Can you work these out from the drawing? Everything is in mm from the part's minimum corner. Round coordinates to 2 decimals unless told otherwise and drop trailing zeros. Order: outer loops, then holes, each group sorted by start corner. A loop starts at its lowest first (then second) coordinate and runs counter-clockwise, first axis right, second up. Notation, with made-up numbers: (75.5, 85) -> (80.5, 85) arc R22 cw to (80.5, 115) -> close; hole circle Ø8 at (47, 56). An arc over 180 degrees is marked (long way). One line per item, written item: value.
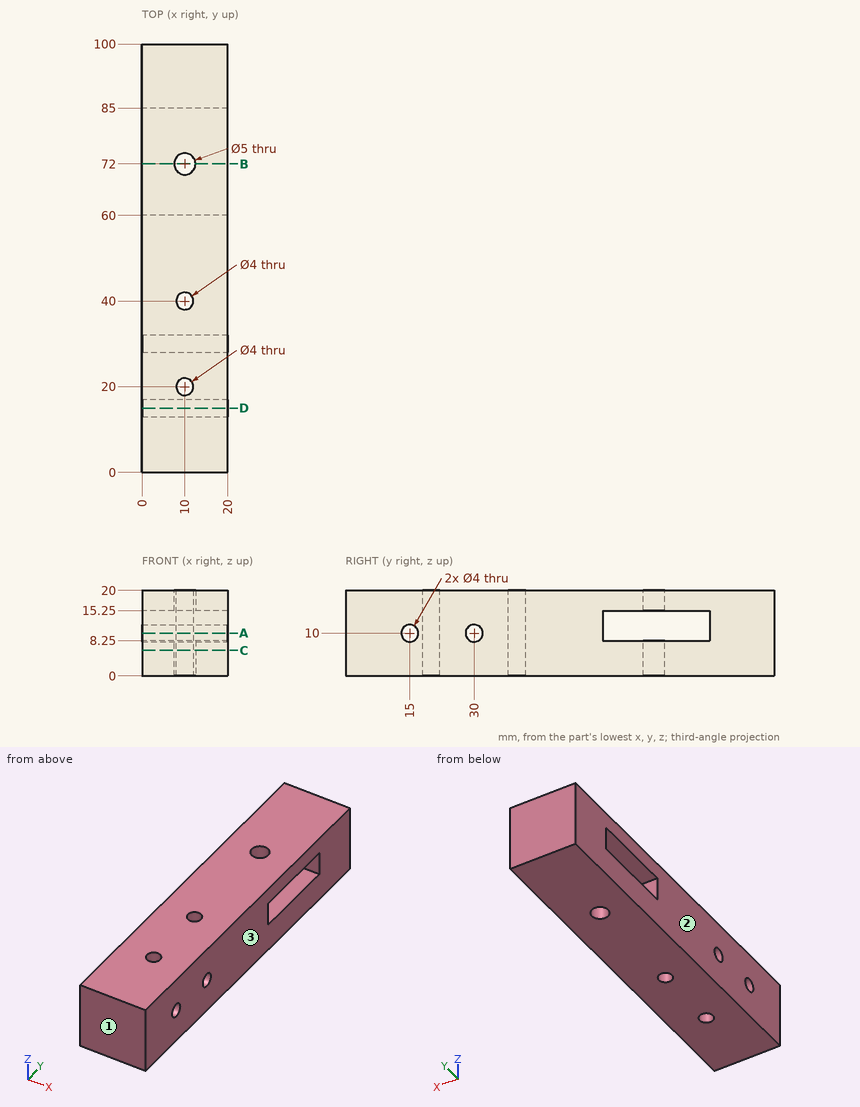
Q1. I want a section at A-A on z = 10. Write out the boundary of the cut face in (x, y).
Answers:
outline: (0, 0) -> (20, 0) -> (20, 13) -> (0, 13) -> close; (0, 17) -> (20, 17) -> (20, 28) -> (0, 28) -> close; (0, 32) -> (20, 32) -> (20, 60) -> (0, 60) -> close; (0, 85) -> (20, 85) -> (20, 100) -> (0, 100) -> close; hole circle Ø4 at (10, 20); hole circle Ø4 at (10, 40)
Q2. I want a section at B-B on y = 72. Write out the boundary of the cut face in (x, z).
Answers:
outline: (0, 0) -> (7.5, 0) -> (7.5, 8.25) -> (0, 8.25) -> close; (0, 15.25) -> (7.5, 15.25) -> (7.5, 20) -> (0, 20) -> close; (12.5, 0) -> (20, 0) -> (20, 8.25) -> (12.5, 8.25) -> close; (12.5, 15.25) -> (20, 15.25) -> (20, 20) -> (12.5, 20) -> close
Q3. I want a section at D-D on y = 15. Write out the boundary of the cut face in (x, z), then the cut area to 3 significant figures.
Answers:
outline: (0, 0) -> (20, 0) -> (20, 8) -> (0, 8) -> close; (0, 12) -> (20, 12) -> (20, 20) -> (0, 20) -> close
area: 320 mm2
Q4. I need wall thicknesses on line 1 along Y through (x, z) = (10, 14.5); line 2 along Y through (x, z) = (10, 17.1); line 3 along Z through (x, y) = (13.5, 15). Which ranges of each line are inside material? Lowest first, please.
Answers:
line 1: 0 to 18, 22 to 38, 42 to 60, 85 to 100
line 2: 0 to 18, 22 to 38, 42 to 69.5, 74.5 to 100
line 3: 0 to 8, 12 to 20
Q5. If we mould it in two halves opening along X, with no side actions, what happens to the marked faces 1, 2 and 3? For each: pulls with the +X half, pulls with the -X half, needs draft (parallel to the pull), parting line crosses it, or undercut.
Answers:
face 1: needs draft
face 2: pulls with the -X half
face 3: pulls with the +X half
Q6. I want a section at C-C on z = 6. Write out the boundary of the cut face in (x, y), then the cut area to 3 significant figures.
Answers:
outline: (0, 0) -> (20, 0) -> (20, 100) -> (0, 100) -> close; hole circle Ø5 at (10, 72); hole circle Ø4 at (10, 20); hole circle Ø4 at (10, 40)
area: 1,960 mm2
